Design review of the part built by this model. Coordinates are the model's own, in mm. A direction names the side the tool comes from. Coordinates: 2 decimals unless noted, no trailing zeros. Loops run counter-clockwise (first coordinate to the right, second up) from the corner with the lowest first, then second, coordinate; pieces in that order, holes last. Notation, with made-up numbers: (72, -1.5) - (125, -1.5) arc R37 ccw to (125, 34.5) - close; hole circle Ø3 at (72.25, 46.25). An arc over 180 degrees is marked (long way). Use one line per item in the form item = value. Start each with the question number.
(1) Add section C-C (y = 19.5). Count the separate pieces of the cut face and the enclosed holes in it, plus the area to 3 significant figures.
(2) Add section D-D (x = 38). State the section outline as (y, z) points, plus the area to 3 significant figures.
(3) Clearance check with flat-ended pins moving along their axes: pin 1 Ø4 at (y, z) = (19.5, 15) entering from -X; pin 2 Ø2.5 at (x, z) = (39.5, 15.5) entering from -Y. State where each tip first meets the part, or that it passes through.
(4) The part is to be moulded in two halves that separate along Z. For faces 1 (the face through (39, 15.5, 15)), 2 (the face through (20.5, 19, 23)), 3 (the face through (40.34, 13.12, 24.8)), say which applies: pulls with the +Z half, pulls with the -Z half, needs draft (parallel to the pull), parting line crosses it, or undercut.
(5) Add section A-A (x = 32.5). State the section outline as (y, z) points, plus the area to 3 significant figures.
(6) Tool access review of faces 4 (the face through (40, 19, 15)), 5 (the face through (29, 17, 9.85)), 6 (the face through (34.5, 25.5, 15.1)): name each direction out of +Z, -Z, +X, -X, +Y, -Y from which nothing blocks a thin tool from reaching the whole face with its end or side.
(7) For L1, parallel to Z at x = 35, y = 17.25; L2, parallel to Y at x = 27.5, z = 6.2; L3, parallel to Y at x = 38, z = 13.5, list the stretches that pass through material, from the lowest coordinate up.
(8) Add section B-B (z = 11.25). State the section outline as (x, y) points.
```python
from build123d import *

# Parameters (mm, degrees)
SKETCH001_W     = 21.5
SKETCH001_H     = 16
PAD_DEPTH       = 20
POCKET_DEPTH    = 6
SKETCH003_R     = 2.45
POCKET001_DEPTH = 20.001
SKETCH004_R     = 4
SKETCH004_R_2   = 2.45
PAD001_DEPTH    = 0.85
SKETCH005_R     = 4
SKETCH005_R_2   = 2.45
PAD002_DEPTH    = 0.85
CHAMFER_SIZE    = 0.84
CHAMFER001_SIZE = 3
CHAMFER002_SIZE = 3
CHAMFER003_SIZE = 0.4
SKETCH010_W     = 10
SKETCH010_H     = 4
POCKET004_DEPTH = 6
SKETCH021_R     = 2.15
POCKET012_DEPTH = 2
CHAMFER010_SIZE = 0.4
CHAMFER011_SIZE = 1


with BuildPart() as part:
    # Sketch001 → Pad (new body)
    with BuildSketch(Plane.XY):
        with Locations((3.75, 0)):
            Rectangle(SKETCH001_W, SKETCH001_H)
    extrude(amount=PAD_DEPTH)

    # Sketch002 (on DatumPlane) → Pocket (cut, symmetric)
    with BuildSketch(Plane.XY.offset(10)):
        Polygon((-7, 8), (5.5, 8), (8.5, 4), (8.5, -4), (5.5, -8), (-7, -8), align=None)
    extrude(amount=POCKET_DEPTH, both=True, mode=Mode.SUBTRACT)

    # Sketch003 (on Face4 of Pocket) → Pocket001 (cut, through all)
    with BuildSketch(Plane.XY.offset(20)):
        Circle(SKETCH003_R)
    extrude(amount=-POCKET001_DEPTH, mode=Mode.SUBTRACT)

    # Sketch004 (on Face8 of Pocket001) → Pad001 (join)
    with BuildSketch(Plane.XY.offset(4)):
        Circle(SKETCH004_R)
        Circle(SKETCH004_R_2, mode=Mode.SUBTRACT)
    extrude(amount=PAD001_DEPTH)

    # Sketch005 (on Face6 of Pad001) → Pad002 (join)
    with BuildSketch(Plane(origin=(0, 0, 16), x_dir=(1, 0, 0), z_dir=(0, 0, -1))):
        Circle(SKETCH005_R)
        Circle(SKETCH005_R_2, mode=Mode.SUBTRACT)
    extrude(amount=PAD002_DEPTH)

    # Chamfer
    chamfer_edges = [part.edges().sort_by_distance(p)[0] for p in [
        (-4, 0, 4.85),
        (-4, 0, 15.15),
    ]]
    chamfer(chamfer_edges, length=CHAMFER_SIZE)

    # Chamfer001
    chamfer001_edges = [part.edges().sort_by_distance(p)[0] for p in [
        (-7, 8, 2),
        (-7, -8, 2),
        (-7, 8, 18),
        (-7, -8, 18),
    ]]
    chamfer(chamfer001_edges, length=CHAMFER001_SIZE)

    # Chamfer002
    chamfer002_edges = [part.edges().sort_by_distance(p)[0] for p in [
        (14.5, -8, 10),
        (14.5, 8, 10),
    ]]
    chamfer(chamfer002_edges, length=CHAMFER002_SIZE)

    # Chamfer003
    chamfer003_edges = [part.edges().sort_by_distance(p)[0] for p in [
        (3.75, 8, 20),
        (13, 6.5, 20),
        (-5.5, 6.5, 20),
        (14.5, 0, 20),
        (-7, 0, 20),
        (13, -6.5, 20),
        (-5.5, -6.5, 20),
        (3.75, -8, 20),
        (-2.45, 0, 20),
        (3.75, 8, 0),
        (13, 6.5, 0),
        (-5.5, 6.5, 0),
        (14.5, 0, 0),
        (-7, 0, 0),
        (13, -6.5, 0),
        (-5.5, -6.5, 0),
        (3.75, -8, 0),
        (-2.45, 0, 0),
    ]]
    chamfer(chamfer003_edges, length=CHAMFER003_SIZE)

    # Sketch010 (on DatumPlane) → Pocket004 (cut, symmetric)
    with BuildSketch(Plane.XY.offset(10)):
        with Locations((9.5, -6)):
            Rectangle(SKETCH010_W, SKETCH010_H)
    extrude(amount=POCKET004_DEPTH, both=True, mode=Mode.SUBTRACT)

    # Sketch021 (on Face10 of Pocket004) → Pocket012 (cut)
    with BuildSketch(Plane.YZ.offset(14.5)):
        with Locations((0, 10)):
            Circle(SKETCH021_R)
    extrude(amount=-POCKET012_DEPTH, mode=Mode.SUBTRACT)

    # Chamfer010
    chamfer010_edges = [part.edges().sort_by_distance(p)[0] for p in [
        (14.5, -2.15, 10),
    ]]
    chamfer(chamfer010_edges, length=CHAMFER010_SIZE)

    # Chamfer011
    chamfer011_edges = [part.edges().sort_by_distance(p)[0] for p in [
        (8.5, -4, 10),
    ]]
    chamfer(chamfer011_edges, length=CHAMFER011_SIZE)


with BuildPart() as part_1:
    # Body001 placement: moved
    add(part.part.moved(Location((27.5, 19.5, 5))))


solid = part_1.part
```
Computed values:
q1.separate_pieces = 3
q1.enclosed_holes = 0
q1.area = 199 mm^2
q2.outline = (11.5, 5.4) - (11.9, 5) - (27.1, 5) - (27.5, 5.4) - (27.5, 24.6) - (27.1, 25) - (11.9, 25) - (11.5, 24.6) - (11.5, 21) - (15.5, 21) - (15.5, 9) - (11.5, 9) - close
q2.area = 272 mm^2
q3.pin_1 = 36
q3.pin_2 = 15.5
q4.face_1 = undercut
q4.face_2 = needs draft
q4.face_3 = pulls with the +Z half
q5.outline = (11.5, 5.4) - (11.9, 5) - (27.1, 5) - (27.5, 5.4) - (27.5, 9) - (11.5, 9) - close; (11.5, 21) - (27.5, 21) - (27.5, 24.6) - (27.1, 25) - (11.9, 25) - (11.5, 24.6) - close
q5.area = 128 mm^2
q6.face_4 = +X
q6.face_5 = -X, +Y, -Y
q6.face_6 = -X, -Y
q7.L1 = 5 to 9, 21 to 25
q7.L2 = 11.5 to 17.05, 21.95 to 27.5
q7.L3 = 15.5 to 27.5
q8.outline = (33, 27.5) - (36, 23.5) - (36, 16.5) - (37, 15.5) - (42, 15.5) - (42, 24.5) - (39, 27.5) - close
